Part print with two shaded views. Sizes in mm from the minimum x, y, z corner. A direction names the side the tool comes from. Give positions to 0.01 mm unless a question says otherwise; leave off trailing zeros. Write each loop counter-clockwise with the first axis right and the second up, starting at its lowest first coordinate (ties: lowest second). Pieces come first, ordered by that corner, then holes. Notation, with made-up numbers: (37.5, 76) -> (96.5, 76) arc R34 cw to (96.5, 109) -> close; hole circle Ø3 at (74, -23). An arc over 180 degrees is marked (long way). Answer as a JSON object with one key per item and string values.
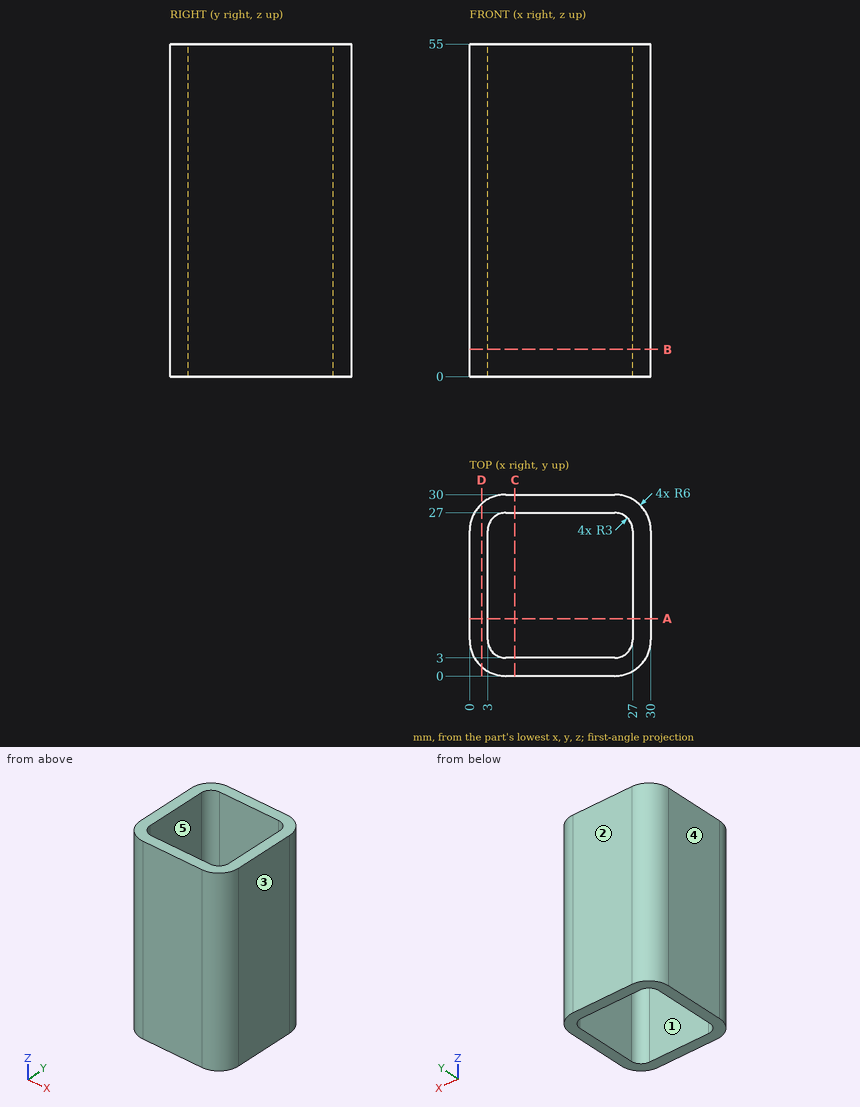
1) 3-axis set-ups, long thin cutter, end or side, ignore diameter. For the marked faces 4 and 5: which of +Z, -Z, +X, -X, +Y, -Y reach the whole face in a straight line?
Model answer:
{"face 4": "+Z, -Z, -X, +Y, -Y", "face 5": "+Z, -Z"}
2) Mould opens along Y. For the marked faces 1, 2 and 3 say: released by +Y, released by -Y, zero draft, split by the parting line, or undercut.
Model answer:
{"face 1": "undercut", "face 2": "released by +Y", "face 3": "zero draft"}
3) Pin check, flat tip, straight feed: pin 1 (4 mm diameter, centred on y = 26.5, z = 8.5, fed in from +X). Stop position of the tip, or through.
Model answer:
{"pin 1": "stops at x = 29.98"}
4) Wall check: probe 1 along X at (y, z) = (23.5, 3.5); probe 2 along Y at (x, z) = (26.75, 14). Give the ranges that are in metal, low to high.
Model answer:
{"probe 1": "x = 0 to 3, 27 to 30", "probe 2": "y = 0.67 to 4.8, 25.2 to 29.33"}
5) Slice it at A-A (y = 9.5). List the corners of the cut face in (x, z).
Model answer:
{"outline": "(0, 0) -> (3, 0) -> (3, 55) -> (0, 55) -> close; (27, 0) -> (30, 0) -> (30, 55) -> (27, 55) -> close"}
6) Slice it at B-B (z = 4.5). List the corners of the cut face in (x, y), then the cut area to 3 significant figures.
Model answer:
{"outline": "(0, 6) arc R6 ccw to (6, 0) -> (24, 0) arc R6 ccw to (30, 6) -> (30, 24) arc R6 ccw to (24, 30) -> (6, 30) arc R6 ccw to (0, 24) -> close; hole (3, 6) arc R3 ccw to (6, 3) -> (24, 3) arc R3 ccw to (27, 6) -> (27, 24) arc R3 ccw to (24, 27) -> (6, 27) arc R3 ccw to (3, 24) -> close", "area": "301 mm2"}
7) Slice it at D-D (x = 2). List the corners of the cut face in (y, z).
Model answer:
{"outline": "(1.53, 0) -> (28.47, 0) -> (28.47, 55) -> (1.53, 55) -> close"}
